from build123d import *

# Parameters (mm, degrees)
SKETCH1_W           = 330.2
SKETCH1_H           = 228.6
BOSS_EXTRUDE1_DEPTH = 6
SKETCH2_R           = 6.25
SKETCH2_R_2         = 3.175
SKETCH2_R_3         = 11
CUT_EXTRUDE1_DEPTH  = 402.654080024


with BuildPart() as part:
    # Sketch1 → Boss-Extrude1 (new body)
    with BuildSketch(Plane(origin=(0, 0, 0), x_dir=(1, 0, 0), z_dir=(0, 1, 0))):
        with Locations((165.1, 114.3)):
            Rectangle(SKETCH1_W, SKETCH1_H)
    extrude(amount=BOSS_EXTRUDE1_DEPTH)

    # Sketch2 → Cut-Extrude1 (cut, through all)
    with BuildSketch(Plane(origin=(0, 6, 0), x_dir=(1, 0, 0), z_dir=(0, 1, 0))):
        with Locations(Location((70.8, 177.6, 0), (0, 0, 270))):
            Circle(SKETCH2_R)
        with Locations(Location((108.9, 173.1, 0), (0, 0, 270))):
            Circle(SKETCH2_R_2)
        with Locations(Location((159.7, 177.6, 0), (0, 0, 270))):
            Circle(SKETCH2_R_2)
        with Locations(Location((207.96, 207.6, 0), (0, 0, 270))):
            Circle(SKETCH2_R_2)
        with Locations(Location((187.5, 139.2, 0), (0, 0, 270))):
            Circle(SKETCH2_R_3)
        with Locations(Location((217.5, 158.6, 0), (0, 0, 270))):
            Circle(SKETCH2_R_3)
        with Locations(Location((255.6, 170.18, 0), (0, 0, 270))):
            Circle(SKETCH2_R_3)
    extrude(amount=-CUT_EXTRUDE1_DEPTH, mode=Mode.SUBTRACT)


solid = part.part
CAD build for the part. Positions are in the model's coordinates, mm. Round coordinates to 2 decimals unless told otherwise and drop trailing zeros. Loops run counter-clockwise (first coordinate to the right, second up) from the corner with the lowest first, then second, coordinate; pieces in that order, holes last. Notation, with made-up numbers: M 85.5,24 L 92.5,24 A26 cw 92.5,45 Z; hole C -31.75,59 d11. An arc over 180 degrees is marked long. One line per question, with ' | ' between items. Start each with the question number.
Item 1: Wall check: line 1 (X direction, y = 1.55, z = -158.6); line 2 (Z direction, x = 159.7, y = 3.65) (3 decimals); line 3 (X direction, y = 3.1, z = -177.6) (3 decimals). Give the ranges that are in metal, low to high.
Item 2: Cut at D-D, the plane x = 251.5. Write the cut outline in (y, z).
Item 3: Cut at B-B, the plane z = -165.5. Write the cut outline in (x, y), plus the area to 3 significant figures.
Item 4: Pin check, flat tip, straight feed: pin 1 Ø5.5 at (x, z) = (108.9, -173.1) entering from -Y. Stop position of the tip, or through.
Item 5: Two-plate mould, pull along X, no slides. Class faces 1 (the cylindrical face through (263.03, 3.04, -178.29)), 2 (the cylindrical face through (211.11, 3.04, -208.01)), 3 (the flat face through (163, 6, -116)): pulls with the +X half, pulls with the -X half, needs draft (parallel to the pull), parting line crosses it, or undercut.
Item 6: Cut at A-A, the plane x = 187.5. Write the cut outline in (y, z), plus the area to 3 significant figures.
Item 7: Cut at C-C, the plane y = 0.95. Write the cut outline in (x, z) (3 decimals).
Responses:
1) line 1: x = 0 to 206.5, 228.5 to 330.2 | line 2: z = -228.6 to -180.775, -174.425 to 0 | line 3: x = 0 to 64.55, 77.05 to 156.525, 162.875 to 247.479, 263.721 to 330.2
2) outline: M 0,-228.6 L 6,-228.6 L 6,-180.39 L 0,-180.39 Z; M 0,-159.97 L 6,-159.97 L 6,0 L 0,0 Z
3) outline: M 0,0 L 208.93,0 L 208.93,6 L 0,6 Z; M 226.07,0 L 245.65,0 L 245.65,6 L 226.07,6 Z; M 265.55,0 L 330.2,0 L 330.2,6 L 265.55,6 Z | area: 1,760 mm²
4) pin 1: passes through
5) face 1: undercut | face 2: undercut | face 3: needs draft
6) outline: M 0,-228.6 L 6,-228.6 L 6,-150.2 L 0,-150.2 Z; M 0,-128.2 L 6,-128.2 L 6,0 L 0,0 Z | area: 1,240 mm²
7) outline: M 0,-228.6 L 330.2,-228.6 L 330.2,0 L 0,0 Z; hole C 70.8,-177.6 d12.5; hole C 108.9,-173.1 d6.35; hole C 159.7,-177.6 d6.35; hole C 187.5,-139.2 d22; hole C 207.96,-207.6 d6.35; hole C 217.5,-158.6 d22; hole C 255.6,-170.18 d22
